```python
from build123d import *

# Parameters (mm, degrees)
F0_W     = 203.2
F0_H     = 152.4
F1_DEPTH = 939.8
F3_DEPTH = 152.401


# Not quite as in the source:
# - a pattern or mirror of a feature is missing from the dataset's text; its kind, count and spacing are read off the source's solid


with BuildPart() as f1:
    # F0 (on Right) → F1 (new body, symmetric)
    with BuildSketch(Plane.YZ):
        Rectangle(F0_W, F0_H)
    extrude(amount=F1_DEPTH, both=True)

    # F2 (on face) → F3 (cut, through all)
    with BuildSketch(Plane.XY.offset(76.2)):
        Polygon((-939.8, 101.6), (-939.8, -101.6), (-855.6318041258, 101.6), align=None)
    f3 = extrude(amount=-F3_DEPTH, mode=Mode.SUBTRACT)

    # F3_copies: F3 across plane
    add(f3.mirror(Plane(origin=(0, 0, 0), x_dir=(0, 0, 1), z_dir=(1, 0, 0))), mode=Mode.SUBTRACT)


solid = f1.part
```
Verification items for the finished model (mm, model axes). Coordinates: 2 decimals unless noted, no trailing zeros. Loops run counter-clockwise (first coordinate to the right, second up) from the corner with the lowest first, then second, coordinate; pieces in that order, holes last. Notation, with made-up numbers: (79, -12.5) - (138, -12.5) arc R18 cw to (138, -0.5) - close; hole circle Ø6 at (61.5, 69.25). An arc over 180 degrees is marked (long way). Return JSON: item names as keys, results as strings.
1. Go/stop test with flat-tipped pins: pin 1 (4 mm diameter, centred on y = -24, z = 20.5, fed in from -X); pin 2 (2 mm diameter, centred on y = 77, z = -43, fed in from -X); pin 3 (6 mm diameter, centred on y = -17, z = 51.5, fed in from -X). Record where each tip stops, or that it passes through.
Established:
{"pin 1": "stops at x = -908.49", "pin 2": "stops at x = -866.24", "pin 3": "stops at x = -906"}
2. Section check B-B, the plane y = -27.5. Record the boundary of the cut face in (x, z), then the cut area to 3 significant figures.
Established:
{"outline": "(-909.11, -76.2) - (909.11, -76.2) - (909.11, 76.2) - (-909.11, 76.2) - close", "area": "277,000 mm2"}
3. Thickness scan on L1, parallel to X at y = 66, z = -40; L2, parallel to X at y = -23.5, z = 29. Record the ranges inside material, lowest first.
Established:
{"L1": "x = -870.38 to 870.38", "L2": "x = -907.45 to 907.45"}
4. Section check A-A, the plane z = -43. Record the boundary of the cut face in (x, y).
Established:
{"outline": "(-939.8, -101.6) - (939.8, -101.6) - (855.63, 101.6) - (-855.63, 101.6) - close"}
